```python
from build123d import *

# Parameters (mm, degrees)
F1_DEPTH       = 52.5
F2_W           = 21.2101023644
F2_H           = 4.993801238
F3_DEPTH       = 5
F5_D           = 5
F5_DEPTH       = 6.1
F5_CBORE_D     = 8.1
F5_CBORE_DEPTH = 3.2
F5_TIP         = 1.5021515476
F6_D           = 5
F6_DEPTH       = 6.1
F6_CBORE_D     = 8.1
F6_CBORE_DEPTH = 3.2
F6_TIP         = 1.5021515476
F7_R           = 2.5
F8_DEPTH       = 15
F9_DEPTH       = 18.5
F11_DEPTH      = 3.5
F13_START      = -3
F12_W          = 16
F12_H          = 15
F13_DEPTH      = 3
F14_START      = -9
F14_DEPTH      = 3
F15_ANGLE      = -90
F18_W          = 25
F18_H          = 18
F19_DEPTH      = 14
F21_R          = 2


with BuildPart() as f1:
    # F0 (on Front) → F1 (new body, symmetric)
    with BuildSketch(Plane.XZ):
        Polygon((-7.7991238795, -1.9758003764), (-7.7991238795, -3.0126834754), (7.814229466, -3.0126834754), (7.814229466, -1.9758003764), (10.6093045324, 0.7892206195), (8.3899200651, 3.0327284253), (-8.4017119181, 3.0327284253), (-10.6092272326, 0.7892206195), align=None)
    extrude(amount=F1_DEPTH, both=True)

    # F2 (on Top) → F3 (cut)
    with BuildSketch(Plane.XY):
        with Locations((0.0056419522, -4.9968052143)):
            Rectangle(F2_W, F2_H)
        with Locations((0.0056419522, -14.9968052143)):
            Rectangle(F2_W, F2_H)
        with Locations((0.0056419522, -24.9968052143)):
            Rectangle(F2_W, F2_H)
        with Locations((0.0056419522, -34.9968052143)):
            Rectangle(F2_W, F2_H)
        with Locations((0.0056419522, -44.9968052143)):
            Rectangle(F2_W, F2_H)
        with Locations((0.0056419522, 5.0031947857)):
            Rectangle(F2_W, F2_H)
        with Locations((0.0056419522, 15.0031947857)):
            Rectangle(F2_W, F2_H)
        with Locations((0.0056419522, 25.0031947857)):
            Rectangle(F2_W, F2_H)
        with Locations((0.0056419522, 35.0031947857)):
            Rectangle(F2_W, F2_H)
        with Locations((0.0056419522, 45.0031947857)):
            Rectangle(F2_W, F2_H)
    extrude(amount=F3_DEPTH, mode=Mode.SUBTRACT)

    # F5
    with Locations(Plane.XY.offset(3.0327284253)):
        with Locations((0, 42.9945960641)):
            CounterBoreHole(F5_D / 2, F5_CBORE_D / 2, F5_CBORE_DEPTH, depth=F5_DEPTH)
            with Locations((0, 0, -(F5_DEPTH + F5_TIP / 2))):  # 118° drill point
                Cone(0, F5_D / 2, F5_TIP, mode=Mode.SUBTRACT)

    # F6
    with Locations(Plane.XY.offset(3.0327284253)):
        with Locations((0, -42.977001518)):
            CounterBoreHole(F6_D / 2, F6_CBORE_D / 2, F6_CBORE_DEPTH, depth=F6_DEPTH)
            with Locations((0, 0, -(F6_DEPTH + F6_TIP / 2))):  # 118° drill point
                Cone(0, F6_D / 2, F6_TIP, mode=Mode.SUBTRACT)


with BuildPart() as f8:
    # F7 (on face) → F8 (new body)
    with BuildSketch(Plane(origin=(0, 0, -3.0126834754), x_dir=(1, 0, 0), z_dir=(0, 0, -1))):
        with BuildLine():
            ThreePointArc((-106.589045567, 38.187250495), (-108.7857447081, 43.4905513539), (-114.089045567, 45.687250495))
            ThreePointArc((-114.089045567, 45.687250495), (-119.3923464259, 43.4905513539), (-121.589045567, 38.187250495))
            ThreePointArc((-121.589045567, 38.187250495), (-119.3923464259, 32.8839496361), (-114.089045567, 30.687250495))
            ThreePointArc((-114.089045567, 30.687250495), (-108.7857447081, 32.8839496361), (-106.589045567, 38.187250495))
        make_face()
        with Locations((-114.089045567, 38.187250495)):
            Circle(F7_R, mode=Mode.SUBTRACT)
        with BuildLine():
            Line((-86.589045567, 45.687250495), (-114.089045567, 45.687250495))
            ThreePointArc((-114.089045567, 45.687250495), (-108.7857447081, 43.4905513539), (-106.589045567, 38.187250495))
            ThreePointArc((-106.589045567, 38.187250495), (-108.7857447081, 32.8839496361), (-114.089045567, 30.687250495))
            Line((-114.089045567, 30.687250495), (-86.589045567, 30.687250495))
            Line((-86.589045567, 30.687250495), (-86.589045567, 45.687250495))
        make_face()
    extrude(amount=F8_DEPTH)

    # F7 (on face) → F9 (join)
    with BuildSketch(Plane(origin=(0, 0, -3.0126834754), x_dir=(1, 0, 0), z_dir=(0, 0, -1))):
        with BuildLine():
            ThreePointArc((-106.589045567, 38.187250495), (-108.7857447081, 43.4905513539), (-114.089045567, 45.687250495))
            ThreePointArc((-114.089045567, 45.687250495), (-119.3923464259, 43.4905513539), (-121.589045567, 38.187250495))
            ThreePointArc((-121.589045567, 38.187250495), (-119.3923464259, 32.8839496361), (-114.089045567, 30.687250495))
            ThreePointArc((-114.089045567, 30.687250495), (-108.7857447081, 32.8839496361), (-106.589045567, 38.187250495))
        make_face()
        with Locations((-114.089045567, 38.187250495)):
            Circle(F7_R, mode=Mode.SUBTRACT)
    extrude(amount=F9_DEPTH)

    # F10 (on face) → F11 (cut)
    with BuildSketch(Plane(origin=(0, 0, -21.5126834754), x_dir=(1, 0, 0), z_dir=(0, 0, -1))):
        Polygon((-111.839045567, 34.2901361779), (-109.589045567, 38.187250495), (-111.839045567, 42.084364812), (-116.339045567, 42.084364812), (-118.589045567, 38.187250495), (-116.339045567, 34.2901361779), align=None)
    extrude(amount=-F11_DEPTH, mode=Mode.SUBTRACT)

    # F12 (on face) → F13 (cut)
    with BuildSketch(Plane.XY.offset(-3.0126834754).offset(F13_START)):
        with Locations((-113.6591356158, -38.187250793)):
            Rectangle(F12_W, F12_H)
    extrude(amount=-F13_DEPTH, mode=Mode.SUBTRACT)

    # F12 (on face) → F14 (cut)
    with BuildSketch(Plane.XY.offset(-3.0126834754).offset(F14_START)):
        with Locations((-113.6591356158, -38.187250793)):
            Rectangle(F12_W, F12_H)
    extrude(amount=-F14_DEPTH, mode=Mode.SUBTRACT)


with BuildPart() as f8_1:
    # F15: moved
    add(f8.part.rotate(Axis((-86.589045567, -38.187250495, -18.0126834754), (0, 1, 0)), F15_ANGLE))


with BuildPart() as f8_2:
    # F16: moved
    add(f8_1.part.moved(Location((94.1, 0, 31))))


with BuildPart() as f8_3:
    # F17: moved
    add(f8_2.part.moved(Location((0, 13.2, 0))))

    # F18 (on face) → F19 (cut)
    with BuildSketch(Plane.XY.offset(12.9873165246)):
        with Locations((0.6974760443, -24.6108990014)):
            Rectangle(F18_W, F18_H)
    extrude(amount=-F19_DEPTH, mode=Mode.SUBTRACT)


with BuildPart() as f1_1:
    add(f1.part)

    # F20: union F8
    add(f8_3.part)

    # F21
    f21_edges = [f1_1.edges().sort_by_distance(p)[0] for p in [
        (0.010954, -32.48725, -3.012683),
        (0.010954, -17.48725, -3.012683),
    ]]
    fillet(f21_edges, radius=F21_R)


solid = f1_1.part
```
Check sheet for the modelled part. Datum: model origin and axes. Units: mm. A direction names the side the tool comes from. Round coordinates to 2 decimals unless told otherwise and drop trailing zeros. Order: outer loops, then holes, each group sorted by start corner. A loop starts at its lowest first (then second) coordinate and runs counter-clockwise, first axis right, second up. Notation, with made-up numbers: (33, -9) - (85, -9) arc R29 ccw to (85, 21) - close; hole circle Ø11 at (75, 61). An arc over 180 degrees is marked (long way). Write item = value, one per line.
Q1. Draft check along X on faces 6 (the face through (9.515, 49.965, 1.895)), 7 (the face through (1.511, -27, -12)), 8 (the face through (0, -35, 0)). Enter one of: pulls with the +X half, pulls with the -X half, needs draft (parallel to the pull), parting line crosses it, or undercut.
Computed:
face_6 = pulls with the +X half
face_7 = undercut
face_8 = needs draft
Q2. Thickness scan on line 1 along Y through (x, z) = (0, -1.25); line 2 along X through (y, z) = (-19.5, -7); line 3 along Z through (x, y) = (1.75, 30). Record the ranges inside material, lowest first.
Computed:
line_1 = -52.5 to -45.48, -40.48 to 40.49, 45.49 to 52.5
line_2 = -7.49 to -4.49, -1.49 to 1.51, 4.51 to 7.51
line_3 = -3.01 to 3.03
Q3. Tool access check on faces 1 (the face through (-0.01, -25.15, -22.01)), 2 (the face through (-8.91, -0.73, -0.88)), 3 (the face through (0, 5, 0)), 4 (the face through (2, -41, -0.167)), 5 (the face through (9.285, -26.909, -11.122)). Record the directions out of +Z, -Z, +X, -X, +Y, -Y that give a thin tool (end or side, any length) a straight path to the whole face; none if there is none.
Computed:
face_1 = -Z, +X, -X
face_2 = -Z, -X, +Y, -Y
face_3 = +Z, +X, -X
face_4 = +Z
face_5 = +X
Q4. Section check B-B (z = -8.25). Record the boundary of the cut face in (x, y).
Computed:
outline = (-7.49, -32.49) - (-4.49, -32.49) - (-4.49, -17.49) - (-7.49, -17.49) - close; (-1.49, -32.49) - (1.51, -32.49) - (1.51, -17.49) - (-1.49, -17.49) - close; (4.51, -32.49) - (7.51, -32.49) - (7.51, -29.11) - (11.01, -29.11) - (11.01, -20.86) - (7.51, -20.86) - (7.51, -17.49) - (4.51, -17.49) - close
Q5. Go/stop test with flat-tipped pins: pin 1 (12 mm diameter, centred on y = -19.5, z = -2, fed in from +X); pin 2 (5 mm diameter, centred on x = 3, z = -11.5, fed in from +Y); pin 3 (4 mm diameter, centred on x = 9.5, z = -14, fed in from -Y); pin 4 (4 mm diameter, centred on y = -13.5, z = -12, fed in from +X). Record where each tip stops, or that it passes through.
Computed:
pin_1 = 10.61
pin_2 = -17.49
pin_3 = -32.49
pin_4 = through
Q6. Section check C-C (x = 0). State how many separate pieces and enclosed holes the cut face has, and give its area (3 significant figures).
Computed:
separate_pieces = 3
enclosed_holes = 1
area = 673 mm^2
